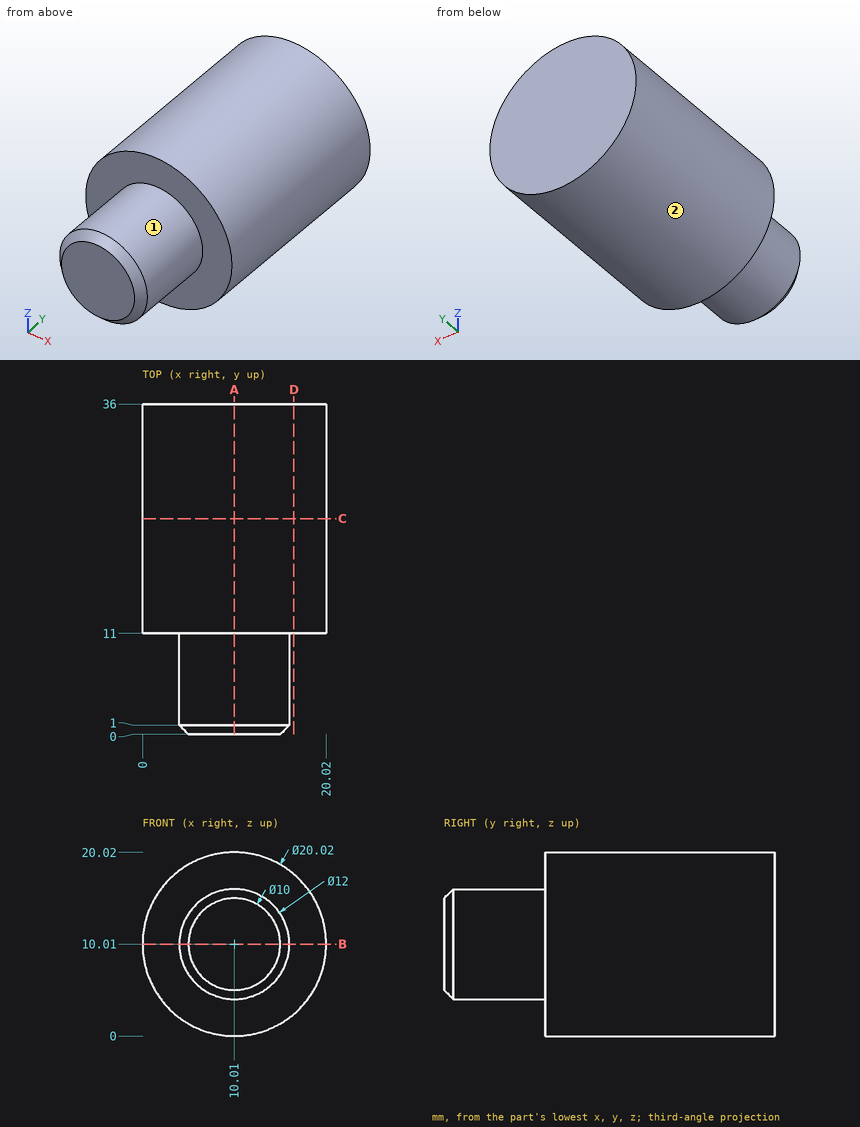
For this review, use the dimensioned drawing (mm, ordinates from the lowest corner) and the shaded views. A direction names the side the tool comes from. Give positions to 0.01 mm unless a question says otherwise; leave off trailing zeros. Order: outer loops, then holes, each group sorted by start corner. A loop starts at its lowest first (then second) coordinate and runs counter-clockwise, first axis right, second up. Notation, with made-up numbers: (40, 37.5) - (52, 37.5) arc R30 ccw to (52, 67.5) - close; hole circle Ø10 at (55.25, 78). An arc over 180 degrees is marked (long way). Write item = value, one per line. Start each with the question number.
Q1. Tool access review of the marked faces 1 and 2: name each direction out of +Z, -Z, +X, -X, +Y, -Y from which nothing blocks a thin tool from reaching the whole face with its end or side.
Q2. We need section A-A on x = 10.01. State the section outline as (y, z) points.
Q3. We need section D-D on x = 16.5. State the section outline as (y, z) points, plus the area to 3 significant figures.
Q4. To check wall thickness, follow L1, parallel to Y at x = 18, z = 5.75; L2, parallel to Z at x = 2, y = 23; L3, parallel to X at y = 29, z = 10.25. State the ranges of each line that lie inside material, in increasing order. Write a range as from..to.
Q5. We need section B-B on z = 10.01. State the section outline as (x, y) points, plus the area to 4 significant figures.
Q6. We need section C-C on y = 23.5. State the section outline as (x, z) points.
Q7. Clearance check with flat-ended pins moving along their axes: pin 1 Ø1.5 at (x, y) = (2.5, 22.5) entering from -Z; pin 2 Ø10 at (y, z) = (29.5, 9) entering from -X; pin 3 Ø1.5 at (x, y) = (4.5, 31.5) entering from -Z; pin 4 Ø5 at (y, z) = (10.5, 17) entering from -X. State where each tip first meets the part, or that it passes through.
Working result:
q1.face_1 = -Y
q1.face_2 = +Y, -Y
q2.outline = (0, 5.01) - (1, 4.01) - (11, 4.01) - (11, 0) - (36, 0) - (36, 20.02) - (11, 20.02) - (11, 16.01) - (1, 16.01) - (0, 15.01) - close
q3.outline = (11, 2.39) - (36, 2.39) - (36, 17.63) - (11, 17.63) - close
q3.area = 381 mm²
q4.L1 = 11..36
q4.L2 = 4.01..16.01
q4.L3 = 0..20.02
q5.outline = (0, 11) - (4.01, 11) - (4.01, 1) - (5.01, 0) - (15.01, 0) - (16.01, 1) - (16.01, 11) - (20.02, 11) - (20.02, 36) - (0, 36) - close
q5.area = 631.5 mm²
q6.outline = circle Ø20.02 at (10.01, 10.01)
q7.pin_1 = 2.63
q7.pin_2 = 0
q7.pin_3 = 1.2
q7.pin_4 = 1.09
